from build123d import *

# Parameters (mm, degrees)
F1_DEPTH = 37.6793125
F2_R     = 6.35
F3_DEPTH = 7.9375


# Not quite as in the source:
# - a pattern or mirror of a feature is missing from the dataset's text; its kind, count and spacing are read off the source's solid


with BuildPart() as f1:
    # F0 (on Front) → F1 (new body, symmetric)
    with BuildSketch(Plane.XZ):
        Polygon((3.6661742094, 6.35), (-3.6661742094, 6.35), (-7.3323484187, 0), (-3.6661742094, -6.35), (3.6661742094, -6.35), (7.3323484187, 0), align=None)
    extrude(amount=F1_DEPTH, both=True)

    # F2 (on face) → F3 (join)
    with BuildSketch(Plane.XZ.offset(37.6793125)):
        Circle(F2_R)
    f3 = extrude(amount=F3_DEPTH)

    # F3_copies: F3 across plane
    add(f3.mirror(Plane.ZX))


solid = f1.part
Here's how the part is built. I have some questions about the finished solid (model axes, mm). A direction names the side the tool comes from. Round coordinates to 2 decimals unless told otherwise and drop trailing zeros. Write each loop counter-clockwise with the first axis right and the second up, starting at its lowest first coordinate (ties: lowest second). Pieces come first, ordered by that corner, then holes.
1. Suppose I cut it at A-A (x = 4.5). List the corners of the cut face in (y, z) for me.
2. Suppose I cut it at C-C (y = 16.5). List the corners of the cut face in (x, z) for me, and give its area (3 significant figures).
3. Suppose I cut it at B-B (z = -1.75). List the corners of the cut face in (x, y) for me.
4. Will these pins go through, and if not, where does the flat tip stop? pin 1 Ø2 at (y, z) = (-27, 1.5) entering from -X; pin 2 Ø2 at (x, y) = (-5, -18.5) entering from +Z.
5. I need wall thicknesses on L1, parallel to Z at x = 5.5, y = 34; L2, parallel to Z at x = -2.25, y = 39.5; L3, parallel to X at y = 40, z = 3.75. Which ranges of each line are inside material? Lowest first, please.
6. For faces 1 (the flat face through (-3, 37.679, 6)), 2 (the flat face through (-3, 37.679, -6)), 3 (the flat face through (3, -37.679, 6)), 4 (the cylindrical face through (-1.38, -41.59, -6.2)), 5 (the flat face through (3, 37.679, 6)), which set-ups out of +Z, -Z, +X, -X, +Y, -Y let a thin tool reach every point of the face, with its end or its side?
Answer sheet:
1. outline: (-45.62, -4.48) - (-37.68, -4.48) - (-37.68, -4.91) - (37.68, -4.91) - (37.68, -4.48) - (45.62, -4.48) - (45.62, 4.48) - (37.68, 4.48) - (37.68, 4.91) - (-37.68, 4.91) - (-37.68, 4.48) - (-45.62, 4.48) - close
2. outline: (-7.33, 0) - (-3.67, -6.35) - (3.67, -6.35) - (7.33, 0) - (3.67, 6.35) - (-3.67, 6.35) - close
2. area: 140 mm2
3. outline: (-6.32, -37.68) - (-6.1, -37.68) - (-6.1, -45.62) - (6.1, -45.62) - (6.1, -37.68) - (6.32, -37.68) - (6.32, 37.68) - (6.1, 37.68) - (6.1, 45.62) - (-6.1, 45.62) - (-6.1, 37.68) - (-6.32, 37.68) - close
4. pin 1: stops at x = -7.04
4. pin 2: stops at z = 5.77
5. L1: z = -3.17 to 3.17
5. L2: z = -5.94 to 5.94
5. L3: x = -5.12 to 5.12
6. face 1: +Z, -X, +Y
6. face 2: -Z, -X, +Y
6. face 3: +Z, +X, -Y
6. face 4: -Y
6. face 5: +Z, +X, +Y
